```python
from build123d import *

# Parameters (mm, degrees)
SKETCH_1_W              = 52
SKETCH_1_H              = 52
EXTRUDE_1_DEPTH         = 31
SKETCH_2_W              = 20.5
SKETCH_2_H              = 52
CUT_EXTRUDE_1_DEPTH     = 20
SKETCH_5_R              = 26
EXTRUDE_2_DEPTH         = 31
CUT_EXTRUDE_2_DEPTH     = 32
SKETCH_7_W              = 20
SKETCH_7_H              = 20.5
CUT_EXTRUDE_3_DEPTH     = 53
EXTRUDE_3_DEPTH         = 27
SKETCH_10_W             = 19
SKETCH_10_H             = 14
SKETCH_11_W             = 19
SKETCH_11_H             = 28
CUT_EXTRUDE_4_DEPTH     = 27
EXTRUDE_4_DEPTH         = 52
SKETCH_13_R             = 2.1
CUT_EXTRUDE_5_DEPTH     = 59
SKETCH_14_R             = 2.1
CUT_EXTRUDE_6_DEPTH     = 48.25
SKETCH_15_R             = 5
CUT_EXTRUDE_7_DEPTH     = 43.2500001
SKETCH_17_W             = 10
SKETCH_17_H             = 42.25
CUT_EXTRUDE_8_DEPTH     = 6.0000001
SKETCH_18_R             = 5
CUT_EXTRUDE_9_DEPTH     = 28.0000001
SKETCH_19_R             = 2.5
CUT_EXTRUDE_10_DEPTH    = 59.0000001
CUT_EXTRUDE1_DEPTH      = 53.0000001
SKETCH3_R               = 7.5
CUT_EXTRUDE2_DEPTH      = 22.300523217
CUT_EXTRUDE2_DEPTH_BACK = 2
CUT_EXTRUDE_12_DEPTH    = 28.0000001
SKETCH_20_W             = 20
SKETCH_20_H             = 14.39
EXTRUDE_5_DEPTH         = 21
CUT_EXTRUDE_11_DEPTH    = 15
FILLET_1_R              = 3


with BuildPart() as part:
    # Эскиз1 → Бобышка-Вытянуть1 (new body)
    with BuildSketch(Plane.XY):
        with Locations((26, 0)):
            Rectangle(SKETCH_1_W, SKETCH_1_H)
    extrude(amount=EXTRUDE_1_DEPTH)

    # Эскиз2 → Вырез-Вытянуть1 (cut)
    with BuildSketch(Plane.ZY):
        with Locations((15.5, 0)):
            Rectangle(SKETCH_2_W, SKETCH_2_H)
    extrude(amount=-CUT_EXTRUDE_1_DEPTH, mode=Mode.SUBTRACT)

    # Эскиз5 → Бобышка-Вытянуть2 (add)
    with BuildSketch(Plane.XY.offset(31)):
        with Locations((41.25, 0)):
            Circle(SKETCH_5_R)
    extrude(amount=-EXTRUDE_2_DEPTH)

    # Эскиз6 → Вырез-Вытянуть2 (cut, through all)
    with BuildSketch(Plane.XY.offset(31)):
        with BuildLine():
            Line((52, 23.673561202), (52, 26))
            Line((52, 26), (25, 26))
            ThreePointArc((25, 26), (38.550021379, 25.417314778), (52, 23.673561202))
        make_face()
    cut_extrude_2 = extrude(amount=-CUT_EXTRUDE_2_DEPTH, mode=Mode.SUBTRACT)

    # Зеркальное отражение1: Вырез-Вытянуть2 across plane
    add(cut_extrude_2.mirror(Plane(origin=(0, 0, 0), x_dir=(0, 0, 1), z_dir=(0, -1, 0))), mode=Mode.SUBTRACT)

    # Эскиз7 → Вырез-Вытянуть3 (cut, through all)
    with BuildSketch(Plane(origin=(0, 26, 0), x_dir=(1, 0, 0), z_dir=(0, 1, 0))):
        with Locations((10, -15.5)):
            Rectangle(SKETCH_7_W, SKETCH_7_H)
    extrude(amount=-CUT_EXTRUDE_3_DEPTH, mode=Mode.SUBTRACT)

    # Эскиз9 → Бобышка-Вытянуть3 (add)
    with BuildSketch(Plane(origin=(0, 0, 0), x_dir=(-1, 0, 0), z_dir=(0, 0, -1))):
        with BuildLine():
            Line((-25, 26), (-25, -26))
            ThreePointArc((-25, -26), (-38.550021379, -25.417314778), (-52, -23.673561202))
            ThreePointArc((-52, -23.673561202), (-67.25, 0), (-52, 23.673561202))
            ThreePointArc((-52, 23.673561202), (-38.550021379, 25.417314778), (-25, 26))
        make_face()
    extrude(amount=EXTRUDE_3_DEPTH)

    # Эскиз10 → Вырез-Повернуть2 (revolve, cut)
    with BuildSketch(Plane.ZY.offset(-41.25)):
        with Locations((-11.25, 7)):
            Rectangle(SKETCH_10_W, SKETCH_10_H)
    revolve(axis=Axis((41.25, 0, -20.75), (0, 0, 1)), mode=Mode.SUBTRACT)

    # Эскиз11 → Вырез-Вытянуть4 (cut, through all)
    with BuildSketch(Plane(origin=(0, 0, 0), x_dir=(0, 0, -1), z_dir=(0, -1, 0))):
        with Locations((11.25, 41.25)):
            Rectangle(SKETCH_11_W, SKETCH_11_H)
    extrude(amount=CUT_EXTRUDE_4_DEPTH, mode=Mode.SUBTRACT)

    # Эскиз12 → Бобышка-Вытянуть4 (add)
    with BuildSketch(Plane.XZ.offset(26)):
        with BuildLine():
            Line((0, 0), (25, 0))
            Line((25, 0), (25, -27))
            ThreePointArc((25, -27), (16.039335617, -10.222837391), (0, 0))
        make_face()
    extrude(amount=-EXTRUDE_4_DEPTH)

    # Эскиз13 → Вырез-Вытянуть5 (cut, through all)
    with BuildSketch(Plane.XY.offset(31)):
        with Locations((10, 0)):
            Circle(SKETCH_13_R)
    extrude(amount=-CUT_EXTRUDE_5_DEPTH, mode=Mode.SUBTRACT)

    # Эскиз14 → Вырез-Вытянуть6 (cut, through all)
    with BuildSketch(Plane.ZY.offset(-20)):
        with Locations((15.5, -21)):
            Circle(SKETCH_14_R)
        with Locations((15.5, 21)):
            Circle(SKETCH_14_R)
    extrude(amount=-CUT_EXTRUDE_6_DEPTH, mode=Mode.SUBTRACT)

    # Эскиз15 → Вырез-Вытянуть7 (cut, through all)
    with BuildSketch(Plane(origin=(25, 0, 0), x_dir=(0, 0, -1), z_dir=(1, 0, 0))):
        with Locations((-15.5, 21)):
            Circle(SKETCH_15_R)
        with Locations((-15.5, -21)):
            Circle(SKETCH_15_R)
    extrude(amount=CUT_EXTRUDE_7_DEPTH, mode=Mode.SUBTRACT)

    # Эскиз17 → Вырез-Вытянуть8 (cut, through all)
    with BuildSketch(Plane(origin=(0, 21, 0), x_dir=(0, 0, -1), z_dir=(0, 1, 0))):
        with Locations((-15.5, -46.125)):
            Rectangle(SKETCH_17_W, SKETCH_17_H)
    cut_extrude_8 = extrude(amount=CUT_EXTRUDE_8_DEPTH, mode=Mode.SUBTRACT)

    # Зеркальное отражение2: Вырез-Вытянуть8 across plane
    add(cut_extrude_8.mirror(Plane(origin=(0, 0, 0), x_dir=(0, 0, 1), z_dir=(0, -1, 0))), mode=Mode.SUBTRACT)

    # Эскиз18 → Вырез-Вытянуть9 (cut, through all)
    with BuildSketch(Plane(origin=(0, 0, 0), x_dir=(-1, 0, 0), z_dir=(0, 0, -1))):
        with Locations((-10, 0)):
            Circle(SKETCH_18_R)
    extrude(amount=CUT_EXTRUDE_9_DEPTH, mode=Mode.SUBTRACT)

    # Эскиз19 → Вырез-Вытянуть10 (cut, through all)
    with BuildSketch(Plane.XY.offset(31)):
        with Locations((41.25, 0)):
            Circle(SKETCH_19_R)
    extrude(amount=-CUT_EXTRUDE_10_DEPTH, mode=Mode.SUBTRACT)


with BuildPart() as body_2:
    # Зеркальное отражение3: mirrored copy
    add(part.part.mirror(Plane.ZY))

    # Sketch1 → Cut-Extrude1 (cut, through all)
    with BuildSketch(Plane(origin=(0, 26, 0), x_dir=(1, 0, 0), z_dir=(0, 1, 0))):
        with BuildLine():
            Line((-67.25, -31), (-25, -31))
            ThreePointArc((-25, -31), (-41.975877859, -10.807868092), (-67.25, -3.25))
            Line((-67.25, -3.25), (-67.25, -31))
        make_face()
    extrude(amount=-CUT_EXTRUDE1_DEPTH, mode=Mode.SUBTRACT)

    # Sketch3 → Cut-Extrude2 (cut, two sides)
    with BuildSketch(Plane.XY.offset(9.699476883)) as cut_extrude2_sk:
        with Locations((-41.25, 0)):
            Circle(SKETCH3_R)
    extrude(amount=CUT_EXTRUDE2_DEPTH, mode=Mode.SUBTRACT)
    extrude(cut_extrude2_sk.sketch, amount=-CUT_EXTRUDE2_DEPTH_BACK, mode=Mode.SUBTRACT)

    # Эскиз23 → Вырез-Вытянуть12 (cut, through all)
    with BuildSketch(Plane(origin=(0, 0, 0), x_dir=(-1, 0, 0), z_dir=(0, 0, -1))):
        with BuildLine():
            Line((10, 5), (0, 5))
            Line((0, 5), (0, -5))
            Line((0, -5), (10, -5))
            Line((10, -5), (15, -5))
            Line((15, -5), (15, 0))
            ThreePointArc((15, 0), (13.535533906, 3.535533906), (10, 5))
        make_face()
    extrude(amount=CUT_EXTRUDE_12_DEPTH, mode=Mode.SUBTRACT)

    # Эскиз20 → Бобышка-Вытянуть5 (add)
    with BuildSketch(Plane.XZ.offset(26)):
        with Locations((-10, -1.945)):
            Rectangle(SKETCH_20_W, SKETCH_20_H)
    extrude(amount=-EXTRUDE_5_DEPTH)

    # Эскиз22 → Вырез-Вытянуть11 (cut)
    with BuildSketch(Plane.XZ.offset(26)):
        Polygon((-10, 1.925426481), (-12.75, 0.33771324), (-12.75, -2.83771324), (-10, -4.425426481), (-7.25, -2.83771324), (-7.25, 0.33771324), align=None)
    extrude(amount=-CUT_EXTRUDE_11_DEPTH, mode=Mode.SUBTRACT)

    # Скругление1
    fillet_1_edges = [body_2.edges().sort_by_distance(p)[0] for p in [
        (0, -15.5, -9.14),
    ]]
    fillet(fillet_1_edges, radius=FILLET_1_R)


solid = body_2.part
```
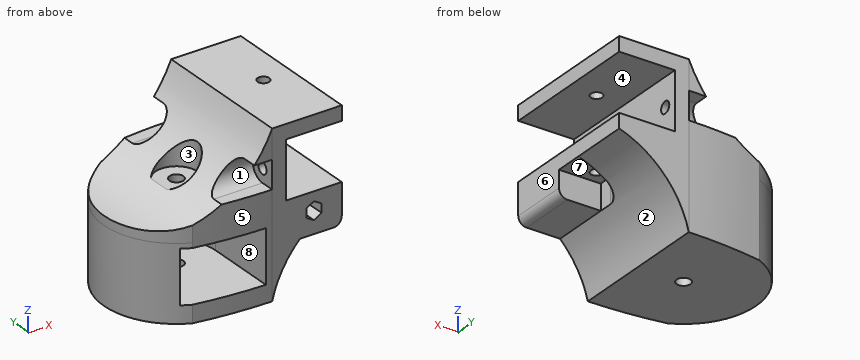
Design review of the part built by this model. Coordinates are the model's own, in mm. Face numbers are marked on the shaded views. A direction names the side the tool comes from. Give positions to 0.01 mm unless a question says otherwise; leave off trailing zeros. Loops run counter-clockwise (first coordinate to the right, second up) from the corner with the lowest first, then second, coordinate; pieces in that order, holes last. Notation, with made-up numbers: (53.25, -4) -> (79.25, -4) arc R19 cw to (79.25, 18) -> close; hole circle Ø9 at (85, 60). An arc over 180 degrees is marked (long way). Write each question's results on one line, items separated by ' | '.
Q1. Machinability: for the marked faces 1, 2, 3 and 4, which of the approach directions +Z, -Z, +X, -X, +Y, -Y give a long, thin tool a straight path to every point of the face, cutting with its end or side? Answer none if there is none.
Reply:
face 1: -X, -Y | face 2: -Z, +X, +Y | face 3: +Z | face 4: +X, +Y, -Y
Q2. Take a section at A-A, the plane y = -10. Write out the cut boundary in (x, z).
Reply:
outline: (-65.25, -27) -> (-25, -27) arc R37.5 cw to (-15, -9.14) -> (-3, -9.14) arc R3 ccw to (0, -6.14) -> (0, 5.25) -> (-20, 5.25) -> (-20, 25.75) -> (0, 25.75) -> (0, 31) -> (-25, 31) arc R46.04 cw to (-65.25, 3.29) -> close; hole (-55.25, -20.75) -> (-27.25, -20.75) -> (-27.25, -1.75) -> (-55.25, -1.75) -> close
Q3. Wall thickness on L1, parallel to Y at x = -20.95, z = 15.5; L2, parallel to Y at x = -10, z = 27; L3, parallel to Y at x = -10, z = 1.4: over which ranges is each line inside the solid? List them lowest first.
Reply:
L1: y = -26 to -23.1, -18.9 to 18.9, 23.1 to 26 | L2: y = -26 to -2.1, 2.1 to 26 | L3: y = -11 to -2.1, 2.1 to 26
Q4. Take a section at C-C, the plane z = 15.5. Write out the cut boundary in (x, y).
Reply:
outline: (-35.98, -16) -> (-25, -16) -> (-25, -18.9) -> (-20, -18.9) -> (-20, 18.9) -> (-25, 18.9) -> (-25, 16) -> (-35.98, 16) -> (-35.98, 5.34) arc R7.5 cw to (-35.98, -5.34) -> close; (-25, -26) -> (-20, -26) -> (-20, -23.1) -> (-25, -23.1) -> close; (-25, 23.1) -> (-20, 23.1) -> (-20, 26) -> (-25, 26) -> close
Q5. Take a section at B-B, the plane x = -41.5. Write out the cut boundary in (y, z), plus the area to 3 significant figures.
Reply:
outline: (-25.14, -27) -> (-2.49, -27) -> (-2.49, -20.75) -> (-25.14, -20.75) -> close; (-25.14, -1.75) -> (-2.49, -1.75) -> (-2.49, 7.7) -> (-7.5, 7.7) -> (-7.5, 11.12) -> (-18.58, 11.12) arc R5 cw to (-21, 10.5) -> (-25.14, 10.5) -> close; (2.49, -27) -> (25.14, -27) -> (25.14, 10.5) -> (21, 10.5) arc R5 cw to (18.58, 11.12) -> (7.5, 11.12) -> (7.5, 7.7) -> (2.49, 7.7) -> (2.49, -1.75) -> (14, -1.75) -> (14, -20.75) -> (2.49, -20.75) -> close | area: 1,040 mm²
Q6. The part is to be moulded in two halves that separate along X. For the marked faces 5, 6, 7 and 8, say which applies: +X half, -X half, draft (parallel to the pull), parting line (faces both ways), or undercut.
Reply:
face 5: -X half | face 6: +X half | face 7: draft | face 8: undercut
Q7. For pin 1 Ø15 at (y, z) = (-8, -7) entering from -X; pin 2 Ø6 at (y, z) = (-14, -12.5) entering from +X; pin 3 Ø4 at (y, z) = (-2, -4) entering from +X, all flat-tipped, find the tip position at first contact; note any pin that passes through.
Reply:
pin 1: stops at x = -67.25 | pin 2: stops at x = -15.35 | pin 3: stops at x = -15
Q8. Take a section at D-D, the plane x = -16.5. Write out the cut boundary in (y, z), plus the area to 3 significant figures.
Reply:
outline: (-26, -10.73) -> (26, -10.73) -> (26, 5.25) -> (-26, 5.25) -> close; (-26, 25.75) -> (26, 25.75) -> (26, 31) -> (-26, 31) -> close | area: 1,100 mm²
